Geometry: final body of the model. Coordinates: model frame, mm. Face numbers are marked on the shaded views. A direction names the side the tool comes from. Give positions to 0.01 mm unless a question says otherwise; leave off trailing zeros. Order: outer loops, then holes, each group sorted by start corner. A loop starts at its lowest first (then second) coordinate and runs counter-clockwise, first axis right, second up. Notation, with made-up numbers: (32.5, 34.5) -> (62.5, 34.5) arc R24 cw to (62.5, 55.5) -> close; hole circle Ø2 at (-22, 29.5). An arc over 180 degrees is marked (long way). One line per question, with ' | ' between items.
from build123d import *

# Parameters (mm, degrees)
BOSS_EXTRUDE1_DEPTH     = 250
FILLET1_R               = 40
SKETCH13_W              = 49.257086068
SKETCH13_H              = 61.833319097
BOSS_EXTRUDE5_DEPTH     = 3
SKETCH14_R              = 5
SKETCH14_R_2            = 4
BOSS_EXTRUDE6_DEPTH     = 50
SKETCH15_R              = 4
CUT_EXTRUDE5_DEPTH      = 50
FILLET5_R               = 10
CUT_EXTRUDE6_DEPTH      = 326.916158871
CUT_EXTRUDE6_DEPTH_BACK = 326.916158871
CUT_EXTRUDE7_DEPTH      = 301.326149824
CUT_EXTRUDE7_DEPTH_BACK = 301.326149824
FILLET6_R               = 50
FILLET7_R               = 50
FILLET8_R               = 50
FILLET9_R               = 50
FILLET10_R              = 50
FILLET11_R              = 100
FILLET12_START          = 43.99041169
FILLET12_DEPTH          = 161.276262689


with BuildPart() as part:
    # Sketch1 → Boss-Extrude1 (new body)
    with BuildSketch(Plane(origin=(0, 0, 0), x_dir=(0, 0, -1), z_dir=(1, 0, 0))):
        Polygon((84.922374429, -7.245973585), (84.922374429, -104.869861266), (7.922374429, -104.869861266), (7.922374429, -107.869861266), (87.922374429, -107.869861266), (87.922374429, -8.272692249), (116.920297026, 29.130138734), (143.207419357, 29.130138734), (143.207419357, 32.130138734), (115.450156075, 32.130138734), align=None)
    extrude(amount=BOSS_EXTRUDE1_DEPTH)

    # Fillet1
    fillet1_edges = [part.edges().sort_by_distance(p)[0] for p in [
        (125, -104.869861266, -84.922374429),
    ]]
    fillet(fillet1_edges, radius=FILLET1_R)

    # Sketch13 → Boss-Extrude5 (add)
    with BuildSketch(Plane(origin=(0, 32.130138734, 0), x_dir=(1, 0, 0), z_dir=(0, 1, 0))):
        with Locations((125, 143.207419358)):
            Rectangle(SKETCH13_W, SKETCH13_H)
    extrude(amount=-BOSS_EXTRUDE5_DEPTH)

    # Sketch14 → Boss-Extrude6 (add)
    with BuildSketch(Plane(origin=(149.628543034, 0, 0), x_dir=(0, 0, -1), z_dir=(1, 0, 0))):
        with Locations((174.124078906, 30.630138734)):
            Circle(SKETCH14_R)
        with Locations((174.124078906, 30.630138734)):
            Circle(SKETCH14_R_2, mode=Mode.SUBTRACT)
    extrude(amount=-BOSS_EXTRUDE6_DEPTH)

    # Sketch15 → Cut-Extrude5 (cut)
    with BuildSketch(Plane(origin=(149.628543034, 0, 0), x_dir=(0, 0, -1), z_dir=(1, 0, 0))):
        with Locations((174.124078906, 30.630138734)):
            Circle(SKETCH15_R)
    extrude(amount=-CUT_EXTRUDE5_DEPTH, mode=Mode.SUBTRACT)

    # Fillet5
    fillet5_edges = [part.edges().sort_by_distance(p)[0] for p in [
        (149.628543034, 30.630138734, -143.207419357),
        (100.371456966, 30.630138734, -143.207419357),
    ]]
    fillet(fillet5_edges, radius=FILLET5_R)

    # Sketch16 → Cut-Extrude6 (cut, two sides: drawn at the far end of the back side and taken through both)
    with BuildSketch(Plane(origin=(0, 0, 0), x_dir=(1, 0, 0), z_dir=(0, 1, 0)).offset(-CUT_EXTRUDE6_DEPTH_BACK)):
        Polygon((152.557475223, 146.136351545), (183.758090757, 115.450156075), (192.952340186, 115.450156075), (215.579344221, 84.922374429), (215.579344221, 35.113164703), (250, 7.922374429), (290.889121347, 148.865149358), (190.317133447, 171.001918434), align=None)
        Polygon((56.304745883, 115.450156075), (65.498995311, 115.450156075), (96.699610846, 146.136351545), (58.939952622, 171.001918434), (-41.632035279, 148.865149358), (-0.742913931, 7.922374429), (33.677741848, 35.113164703), (33.677741848, 84.922374429), align=None)
    extrude(amount=CUT_EXTRUDE6_DEPTH + CUT_EXTRUDE6_DEPTH_BACK, mode=Mode.SUBTRACT)

    # Sketch20 → Cut-Extrude7 (cut, two sides: drawn at the far end of the back side and taken through both)
    with BuildSketch(Plane(origin=(215.579344221, 0, 0), x_dir=(0, 0, -1), z_dir=(1, 0, 0)).offset(-CUT_EXTRUDE7_DEPTH_BACK)):
        Polygon((7.922374429, -107.869861266), (53.377825638, -106.568275865), (64.247416618, -99.891893537), (2.905628415, -97.28009186), (4.033474998, -102.693755458), align=None)
    extrude(amount=CUT_EXTRUDE7_DEPTH + CUT_EXTRUDE7_DEPTH_BACK, mode=Mode.SUBTRACT)

    # Fillet6
    fillet6_edges = [part.edges().sort_by_distance(p)[0] for p in [
        (124.628543034, -7.245973585, -84.922374429),
    ]]
    fillet(fillet6_edges, radius=FILLET6_R)

    # Fillet7
    fillet7_edges = [part.edges().sort_by_distance(p)[0] for p in [
        (124.628543034, -8.272692249, -87.922374429),
    ]]
    fillet(fillet7_edges, radius=FILLET7_R)

    # Fillet8
    fillet8_edges = [part.edges().sort_by_distance(p)[0] for p in [
        (124.628543034, 29.130138734, -116.920297026),
    ]]
    fillet(fillet8_edges, radius=FILLET8_R)

    # Fillet9
    # the kernel refuses this fillet: 50 mm, written as the material it takes off along each edge
    with BuildSketch(Plane(origin=(192.952340186, -29.84551843, -115.450156075), x_dir=(0.5954625750047567, 0, 0.8033830479719526), z_dir=(0, 1, 0))) as fillet9_piece_1:
        with BuildLine():
            CenterArc((20.680282204, -50), FILLET9_R, 90, 31.540576836)
            Line((-5.47483144, -7.38650413), (0, 0))
            Line((0, 0), (20.680282204, 0))
        make_face()
    extrude(amount=113.676362673, mode=Mode.SUBTRACT)

    # Fillet10
    # the kernel refuses this fillet: 50 mm, written as the material it takes off along each edge
    with BuildSketch(Plane(origin=(56.304745883, 83.830844243, -115.450156075), x_dir=(-0.5954625750047574, 0, 0.8033830479719519), z_dir=(0, -1, 0))) as fillet10_piece_1:
        with BuildLine():
            CenterArc((20.680282204, -50), FILLET10_R, 90, 31.540576836)
            Line((-5.47483144, -7.38650413), (0, 0))
            Line((0, 0), (20.680282204, 0))
        make_face()
    extrude(amount=113.676362673, mode=Mode.SUBTRACT)

    # Fillet11
    fillet11_edges = [part.edges().sort_by_distance(p)[0] for p in [
        (65.498995311, 26.992662907, -115.450156075),
        (183.758090757, 26.992662907, -115.450156075),
    ]]
    fillet(fillet11_edges, radius=FILLET11_R)

    # Fillet12: read off the stored shape, not the designer's step
    # Fillet12 outline → Fillet12 (cut)
    with BuildSketch(Plane.YZ.offset(FILLET12_START)):
        with BuildLine():
            Line((29.130138734, -113.124295559), (16.638670002, -103.439824252))
            ThreePointArc((16.638670002, -103.439824252), (28.049083949, -117.450064663), (32.130138734, -135.052035423))
            Line((32.130138734, -135.052035423), (32.130138734, -112.290759809))
            Line((32.130138734, -112.290759809), (29.130138734, -112.290759809))
            Line((29.130138734, -112.290759809), (29.130138734, -113.124295559))
        make_face()
    extrude(amount=FILLET12_DEPTH, mode=Mode.SUBTRACT)


solid = part.part
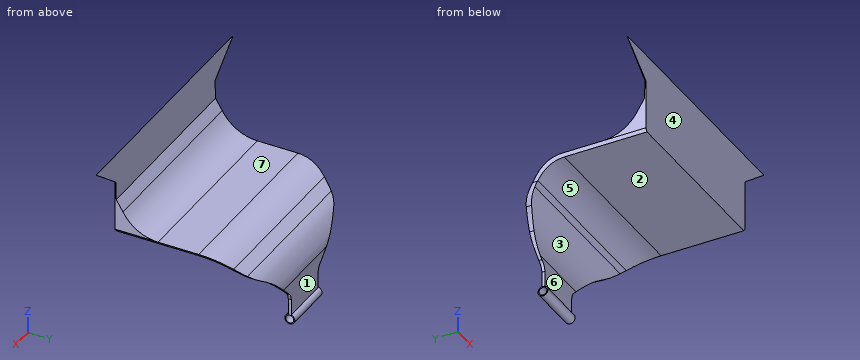
1) Section C-C on x = 71.5. Return loops of the section in (y, z), plus the area to 3 significant figures.
Check result:
outline: (-107.87, -87.92) -> (-25.38, -87.92) arc R50 cw to (5.25, -98.41) -> (9.77, -101.91) arc R50 cw to (25.03, -121.6) -> (29.8, -121.6) arc R40 ccw to (16.64, -103.44) -> (6.28, -95.41) arc R50 ccw to (-24.36, -84.92) -> (-64.87, -84.92) arc R40 cw to (-99.89, -64.25) -> (-106.57, -53.38) -> (-107.87, -7.92) -> close | area: 931 mm^2
2) Material intervals for probe 1 along Z at (x, y) = (150.5, -49); probe 2 along Z at (x, y) = (186, 1.5); probe 3 along Y at (x, z) = (93, -19), sorted ascending. Write a range as from..to.
Check result:
probe 1: z = -87.92..-84.92 | probe 2: z = -95.77..-92.13 | probe 3: y = -107.87..-107.55
3) Section B-B on y = -92. Return loops of the section in (x, z).
Check result:
outline: (33.68, -84.92) -> (35.9, -87.92) -> (213.36, -87.92) -> (215.58, -84.92) -> (215.58, -74.32) -> (33.68, -74.32) -> close
4) Contact query for flat-ended pins moving along their axis: pin 1 Ø8 at (x, y) = (134.5, 18.5) entering from -Z; pin 2 Ø8 at (x, z) = (119.5, -112.5) entering from -Y; pin 3 Ø3 at (y, z) = (30.5, -169) entering from +X; pin 4 Ø21.5 at (y, z) = (-80, -57) entering from +X. Output: stop coordinate, or through.
Check result:
pin 1: stops at z = -116.54 | pin 2: stops at y = 16.76 | pin 3: stops at x = 149.63 | pin 4: passes through
5) Section D-D on z = -26. Return loops of the section in (x, y), plus the area to 3 significant figures.
Check result:
outline: (22.14, -107.87) -> (227.12, -107.87) -> (227.12, -107.35) -> (22.14, -107.35) -> close | area: 106 mm^2
6) Pull-direction query (Z, two-part tool) for the marked faces 4, 5, 6 and 7; classes: +Z half, -Z half, draft (parallel to the pull), parting line (faces both ways), or undercut.
Check result:
face 4: draft | face 5: -Z half | face 6: undercut | face 7: +Z half
7) Section A-A on x = 107. Return loops of the section in (y, z).
Check result:
outline: (-107.87, -87.92) -> (-25.38, -87.92) arc R50 cw to (5.25, -98.41) -> (9.77, -101.91) arc R50 cw to (29.13, -141.42) -> (29.13, -169.35) arc R5 ccw (long way) to (32.13, -169.35) -> (32.13, -135.05) arc R40 ccw to (16.64, -103.44) -> (6.28, -95.41) arc R50 ccw to (-24.36, -84.92) -> (-64.87, -84.92) arc R40 cw to (-99.89, -64.25) -> (-106.57, -53.38) -> (-107.87, -7.92) -> close; hole circle Ø8 at (30.63, -174.12)
8) Set-up query: the marked faces 1, 2 and 3. Return all of +Z, -Z, +X, -X, +Y, -Y with unobstructed straight access to the full face (end or side cutting, diameter ignored); none if empty.
Check result:
face 1: +Z, +X, -X, +Y | face 2: -Z, +X, -X, -Y | face 3: +X, -X, -Y
